Work out the finished part from the listing and answer in its coordinate system (mm). Face numbers are marked on the shaded views. A direction names the side the tool comes from. Give positions to 0.01 mm unless a question says otherwise; leave off trailing zeros. Loops run counter-clockwise (first coordinate to the right, second up) from the corner with the lowest first, then second, coordinate; pieces in that order, holes last. Notation, with made-up numbers: (57.5, 34) - (96.5, 34) arc R23 ccw to (96.5, 66) - close; hole circle Ø3 at (-16, 13). An arc over 180 degrees is marked (long way). One line per question, with ' | ' between items. Start each with the question number.
1. Section D-D (x = -8.5) is taken. Determine the outline of the cut face in (y, z).
2. Find the intervals of material crossed by line 1 (Y direction, x = -3.5, z = 28); line 2 (Y direction, x = 0, z = 26); line 3 (X direction, y = -4, z = 52), in increasing order.
3. Section C-C (x = -2) is taken. Determine the outline of the cut face in (y, z), plus the area to 3 significant figures.
4. Section A-A (z = 5) is taken. Determine the outline of the cut face in (x, y), plus the area to 3 significant figures.
5. Section B-B (y = 0) is taken. Determine the outline of the cut face in (x, z), plus the area to 3 significant figures.
6. For a pull along X with two mould halves and no side action, classify the marked faces 1, 2 and 3 as released by +X, released by -X, zero draft, split by the parting line, or undercut.
7. Each of these flat-tipped pins is pushed along its axis until it touches: pin 1 (2 mm diameter, centred on x = -3.5, y = -14, fed in from -Z); pin 2 (7 mm diameter, centred on x = -3.5, z = 48.5, fed in from -Y); pin 3 (3 mm diameter, centred on x = -7.5, z = 12.5, fed in from +Y); pin 4 (3 mm diameter, centred on x = -1, z = 39.5, fed in from -Y). Where does it stop, or does it pass through?
8. Which of the six approach directions +Z, -Z, +X, -X, +Y, -Y give full straight-line access (tool end or side, diameter ignored) to the marked faces 4, 5 and 6?
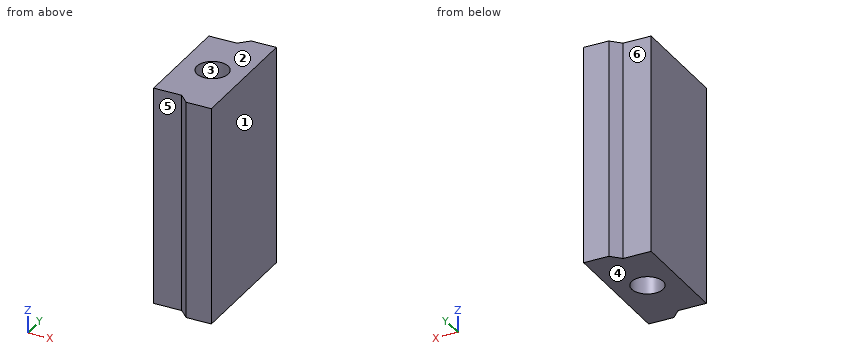
from build123d import *

# Parameters (mm, degrees)
SKETCH_1_W          = 20
SKETCH_1_H          = 39.865713352
EXTRUDE_1_DEPTH     = 70
CUT_EXTRUDE_1_DEPTH = 70
SKETCH_3_R          = 5
CUT_EXTRUDE_2_DEPTH = 74.466446595


with BuildPart() as part:
    # 草图1 → 凸台-拉伸1 (new body)
    with BuildSketch(Plane.XY):
        Rectangle(SKETCH_1_W, SKETCH_1_H)
    extrude(amount=EXTRUDE_1_DEPTH)

    # 草图2 → 切除-拉伸1 (cut)
    with BuildSketch(Plane.XY.offset(70)):
        Polygon((-10, -19.932856676), (1.964722344, -19.932856676), (-1.035277656, -16.932856676), (-10, -16.932856676), align=None)
        Polygon((-10, 19.932856676), (-10, 16.932856676), (-1.035277656, 16.932856676), (1.964722344, 19.932856676), align=None)
    extrude(amount=-CUT_EXTRUDE_1_DEPTH, mode=Mode.SUBTRACT)

    # 草图3 → 切除-拉伸2 (cut, through all)
    with BuildSketch(Plane.XY.offset(70)):
        Circle(SKETCH_3_R)
    extrude(amount=-CUT_EXTRUDE_2_DEPTH, mode=Mode.SUBTRACT)


solid = part.part
Conclusion:
1) outline: (-16.93, 0) - (16.93, 0) - (16.93, 70) - (-16.93, 70) - close
2) line 1: -16.93 to -3.57, 3.57 to 16.93 | line 2: -17.97 to -5, 5 to 17.97 | line 3: -10 to -3, 3 to 10
3) outline: (-16.93, 0) - (-4.58, 0) - (-4.58, 70) - (-16.93, 70) - close; (4.58, 0) - (16.93, 0) - (16.93, 70) - (4.58, 70) - close | area: 1,730 mm²
4) outline: (-10, -16.93) - (-1.04, -16.93) - (1.96, -19.93) - (10, -19.93) - (10, 19.93) - (1.96, 19.93) - (-1.04, 16.93) - (-10, 16.93) - close; hole circle Ø10 at (0, 0) | area: 656 mm²
5) outline: (-10, 0) - (-5, 0) - (-5, 70) - (-10, 70) - close; (5, 0) - (10, 0) - (10, 70) - (5, 70) - close | area: 700 mm²
6) face 1: released by +X | face 2: zero draft | face 3: undercut
7) pin 1: z = 0 | pin 2: y = -17.97 | pin 3: y = 16.93 | pin 4: y = -18.47
8) face 4: -Z, +X, -X, +Y, -Y | face 5: +Z, -Z, -X, -Y | face 6: +Z, -Z, -X, +Y
